Model file for the job. Use its own axes, mm. A direction names the side the tool comes from. Give positions to 0.01 mm unless a question says otherwise; leave off trailing zeros. Loops run counter-clockwise (first coordinate to the right, second up) from the corner with the lowest first, then second, coordinate; pieces in that order, holes last. Notation, with made-up numbers: M -35.5,39 L -0.5,39 A31 cw -0.5,76 Z; hole C 65,-12.5 d1. An arc over 180 degrees is marked long. Use CSV: the item, a comma, the result in double quotes. Start each with the question number.
(1) Slice it at C-C on y = -1.75. List the corners of the cut face in (x, z), and give its area (3 significant figures).
(2) Slice it at B-B on y = 0.45. List the corners of the cut face in (x, z), and give its area (3 significant figures).
(3) Slice it at A-A on z = 0.45. List the corners of the cut face in (x, y), and give its area (3 significant figures).
(4) Wall check: line 1 along X through (y, z) = (-0.75, 0.8); line 2 along Y through (x, z) = (-2.1, 0.3); line 3 along X through (y, z) = (3, 0.9). Give the ranges that are in metal, low to high. Write a range as from..to.
(5) Tool access for faces 1 (the face through (-2.4, 0.5, 0.5)), 2 (the face through (2.4, 0.5, 0.5)), 3 (the face through (0, 0, 0)): list every direction of +Z, -Z, +X, -X, +Y, -Y with a clear straight run to the whole face (end or side of a thin tool).
```python
from build123d import *

# Parameters (mm, degrees)
F0_W     = 4.8
F0_H     = 5
F1_DEPTH = 1
F2_R     = 1


with BuildPart() as f1:
    # F0 (on Top) → F1 (new body)
    with BuildSketch(Plane.XY):
        with BuildLine():
            Line((-2.4, 2.5), (2.4, 2.5))
            ThreePointArc((2.4, 2.5), (2.8, 2.9), (2.4, 3.3))
            Line((2.4, 3.3), (0, 3.3))
            Line((0, 3.3), (-2.4, 3.3))
            ThreePointArc((-2.4, 3.3), (-2.8, 2.9), (-2.4, 2.5))
        make_face()
        Rectangle(F0_W, F0_H)
    extrude(amount=F1_DEPTH)

    # F2
    f2_edges = [f1.edges().sort_by_distance(p)[0] for p in [
        (-2.4, -2.5, 0.5),
        (2.4, -2.5, 0.5),
    ]]
    fillet(f2_edges, radius=F2_R)


solid = f1.part
```
Reply:
1,outline,"M -2.37,0 L 2.37,0 L 2.37,1 L -2.37,1 Z"
1,area,"4.74 mm^2"
2,outline,"M -2.4,0 L 2.4,0 L 2.4,1 L -2.4,1 Z"
2,area,"4.80 mm^2"
3,outline,"M -2.4,-1.5 A1 ccw -1.4,-2.5 L 1.4,-2.5 A1 ccw 2.4,-1.5 L 2.4,2.5 A0.4 ccw 2.4,3.3 L -2.4,3.3 A0.4 ccw -2.4,2.5 Z"
3,area,"27.9 mm^2"
4,line 1,"x = -2.4..2.4"
4,line 2,"y = -2.21..3.3"
4,line 3,"x = -2.79..2.79"
5,face 1,"+Z, -Z, -X, -Y"
5,face 2,"+Z, -Z, +X, -Y"
5,face 3,"-Z, +X, -X, +Y, -Y"
